The listing builds one solid part. Answer for the finished solid, in the listing's coordinates (mm). Face numbers are marked on the shaded views. A direction names the side the tool comes from. Coordinates: 2 decimals unless noted, no trailing zeros. Order: outer loops, then holes, each group sorted by start corner. A loop starts at its lowest first (then second) coordinate and runs counter-clockwise, first axis right, second up. Notation, with made-up numbers: (14.25, 28.25) -> (45.25, 28.25) arc R28 ccw to (45.25, 65.25) -> close; hole circle Ø2 at (60, 23.5). An arc over 180 degrees is marked (long way). Answer in a Markdown table with one row per item.
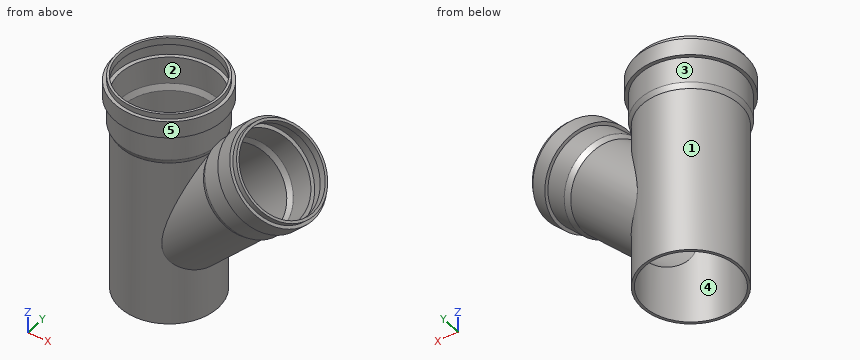
Autodesk Inventor part; units mm, degrees
ref_plane "YZ Plane" through (0, 0, 0) normal (1, 0, 0) x (0, 1, 0)
ref_plane "XZ Plane" through (0, 0, 0) normal (0, 1, 0) x (-1, 0, 0)
ref_plane "XY Plane" through (0, 0, 0) normal (0, 0, 1) x (1, 0, 0)
sketch "Sketch1" plane through (0, 0, 0) normal (0, 1, 0) x (-1, 0, 0)
  line L0 (0, 0) -> (0, 283.8404)
  line L1 (-65.58, 222.1797) -> (-62.5, 215.8203)
  line L2 (-65.58, 283.8404) -> (-62.7, 283.8404)
  line L3 (-62.7, 222.8404) -> (-59.3, 215.8203)
  line L4 (0, 0) -> (-62.5, 0) construction
  line L5 (-59.3, 215.8203) -> (-59.3, 0)
  line L6 (-62.5, 215.8203) -> (-62.5, 0)
  line L7 (-59.3, 0) -> (-62.5, 0)
  line L8 (-62.7, 283.8404) -> (0, 283.8404) construction
  line L9 (-62.5, 0) -> (-59.3, 0)
  line L10 (-64.04, 219) -> (0, 219) construction
  line L11 (0, 78) -> (-62.5, 78) construction
  line L12 (0, 60) -> (-62.5, 60) construction
  line L13 (0, 78) -> (-145.3176, 223.3176)
  line L14 (0, 78) -> (-36.6281, 41.3719) construction
  line L15 (-36.6281, 41.3719) -> (-135.9695, 140.7133)
  line L16 (-36.6281, 41.3719) -> (-38.8909, 39.1091) construction
  line L17 (-38.8909, 39.1091) -> (-138.2323, 138.4505)
  line L18 (-36.6281, 41.3719) -> (-38.8909, 39.1091)
  line L19 (-135.9695, 140.7133) -> (-143.3377, 143.2731)
  line L20 (-184.3499, 184.2853) -> (-186.6126, 182.0225)
  line L21 (-145.6004, 141.0103) -> (-138.2323, 138.4505)
  line L22 (-141.9163, 139.7304) -> (-101.8234, 179.8234) construction
  line L23 (-65.58, 222.1797) -> (-65.58, 255.4404)
  line L24 (-65.58, 255.4404) -> (-69.9, 255.4404)
  line L25 (-69.9, 255.4404) -> (-69.9, 277.1404)
  line L26 (-69.9, 277.1404) -> (-65.58, 277.1404)
  line L27 (-65.58, 277.1404) -> (-65.58, 283.8404)
  line L28 (-62.7, 283.8404) -> (-62.7, 274.7404)
  line L29 (-62.7, 274.7404) -> (-67.5, 274.7404)
  line L30 (-67.5, 274.7404) -> (-67.5, 257.8404)
  line L31 (-67.5, 257.8404) -> (-62.7, 257.8404)
  line L32 (-62.7, 257.8404) -> (-62.7, 222.8404)
  line L33 (-143.3377, 143.2731) -> (-165.9651, 165.9005)
  line L34 (-165.9651, 165.9005) -> (-169.3592, 162.5064)
  line L35 (-169.3592, 162.5064) -> (-181.3093, 174.4565)
  line L36 (-181.3093, 174.4565) -> (-177.9152, 177.8506)
  line L37 (-184.3499, 184.2853) -> (-177.9152, 177.8506)
  line L38 (-186.6126, 182.0225) -> (-181.875, 177.2849)
  line L39 (-181.875, 177.2849) -> (-184.7034, 174.4565)
  line L40 (-184.7034, 174.4565) -> (-169.3592, 159.1123)
  line L41 (-169.3592, 159.1123) -> (-166.5308, 161.9407)
  line L42 (-166.5308, 161.9407) -> (-145.6004, 141.0103)
  line L43 (-184.3499, 184.2853) -> (-145.3176, 223.3176) construction
  line L44 (-135.9695, 140.7133) -> (-99.3414, 177.3414) construction
  line L45 (-143.3377, 143.2731) -> (-104.3054, 182.3054) construction
  line L46 (-62.5, 215.8203) -> (-59.3, 215.8203) construction
  line L47 (-62.7, 222.8404) -> (0, 222.8404) construction
  dimension "d0" = 125
  dimension "d1" = 3.2
  dimension "d2" = 60
  dimension "d3" = 18
  dimension "d4" = 141
  dimension "d5" = 45
  dimension "d6" = 110
  dimension "d7" = 3.2
  dimension "d8" = 144
  dimension "d12" = 125.4
  dimension "d13" = 2.4
  dimension "d14" = 2.4
  dimension "d15" = 2.4
  dimension "d16" = 26
  dimension "d17" = 7.2
  dimension "d18" = 2.88
  dimension "d19" = 2.4
  dimension "d20" = 2.4
  dimension "d21" = 2.4
  dimension "d22" = 7.2
  dimension "d23" = 26
  dimension "d24" = 110.4
  dimension "d25" = 9.1
  dimension "d26" = 2.88
  dimension "d27" = 35
  dimension "d28" = 2.88
  dimension "d29" = 9.1
  dimension "d30" = 32
revolve "Revolution1" add sketch "Sketch1" angle 360 about axis through (0, 0, 0) along (0, 0, 1) contours L23 L24 L25 L26 L27 L2 L28 L29 L30 L31 L32 L3 L5 L13 L6 L1 | L13 L5 L15 L6 | L15 L5 L17 L6 | L17 L5 L7 L6
revolve "Revolution2" add sketch "Sketch1" angle 360 about axis through (0, 0, 78) along (0.7071, 0, 0.7071) contours L15 L5 L17 L6 | L6 L17 L21 L42 L41 L40 L39 L38 L20 L37 L36 L35 L34 L33 L19 L15 | L15 L18 L17 L5
sketch "Sketch2" plane through (145.3176, 0, 223.3176) normal (0.7071, 0, 0.7071) x (0.7071, 0, -0.7071)
  circle A0 centre (0, 0) radius 55.2
  circle A1 centre (0, 0) radius 51.8
  arc A2 (-16.8261, -2.4255) -> (-16.8261, 2.4255) centre (0, 0) ccw
sketch "Sketch3" plane through (0, 0, 283.8404) normal (0, 0, 1) x (1, 0, 0)
  circle A0 centre (0, 0) radius 62.7
  circle A1 centre (0, 0) radius 59.3
  arc A2 (34.4837, 1.0611) -> (34.4837, -1.0611) centre (0, 0) ccw
extrude "Extrusion1" cut sketch "Sketch3" against normal through all contours A1
extrude "Extrusion2" cut sketch "Sketch2" against normal up to surface contours A1
equation "\"d0\" = De"
equation "\"d2\" = L1"
equation "\"d3\" = z1"
equation "\"d12\" = Ds"
equation "\"d13\" = e3"
equation "\"d10\" = L1 + z2"
equation "\"De\" = 125"
equation "\"Ds\" = 125.4"
equation "\"L1\" = 60"
equation "\"e\" = 3.2"
equation "\"z1\" = 18"
equation "\"z2\" = 144"
equation "\"z3\" = 141"
equation "\"e2\" = 0.9 * e"
equation "\"e3\" = 0.75 * e"
equation "\"A\" = 35"
equation "\"C1\" = 26"
equation "\"C2\" = 26"
equation "\"A1\" = 32"
equation "\"e1\" = 3.2"
equation "\"e12\" = 2.88"
equation "\"e13\" = 2.4"
equation "\"L2\" = 54"
equation "\"Ds1\" = 110.4"
equation "\"Size_Designation\" = 1.2345"
properties part number "ISO 3633 45 Deg Reducing Branch with Single Socket for Elastomeric Sealing Ring Joints DN125 x DN110" material "PVC, Unplasticized"
(1) Which of the six approach directions +Z, -Z, +X, -X, +Y, -Y give full straight-line access (tool end or side, diameter ignored) to the marked faces 3, 4 and 5?
Check values:
| item | result |
|---|---|
| face 3 | none |
| face 4 | +Z, -Z |
| face 5 | +Z |
(2) For a pull along Y with two mould halves and no side action, classify the marked faces 1 and 2 as released by +Y, released by -Y, zero draft, split by the parting line, or undercut.
Check values:
| item | result |
|---|---|
| face 1 | split by the parting line |
| face 2 | undercut |
(3) Find the intervals of material crossed by line 1 along Y through (x, z) = (0, 265); line 2 along Y through (x, z) = (0, 246.5); line 3 along Z through (x, y) = (59.5, 27), in increasing order. Write a range as from..to.
Check values:
| item | result |
|---|---|
| line 1 | -69.9..-67.5, 67.5..69.9 |
| line 2 | -65.58..-62.7, 62.7..65.58 |
| line 3 | 69.74..74.98, 200.02..205.26, 221.68..257.84, 274.74..283.84 |
(4) Flat-ended cylindrical pins translate along their axes: pin 1 (2 mm diameter, centred on x = 9, z = 170.5, fed in from +Y); pin 2 (10 mm diameter, centred on y = 23, z = 213, fed in from +X); pin 3 (2 mm diameter, centred on y = 53, z = 76.5, fed in from +X). Find the tip coordinate at first contact, or state that the pin passes through.
Check values:
| item | result |
|---|---|
| pin 1 | y = 61.99 |
| pin 2 | x = 70.19 |
| pin 3 | x = 34.67 |
(5) A cutting plane is placed at C-C, the plane y = 40. Count the separate pieces of the cut face and the enclosed holes in it, then the cut area to 3 significant figures.
Check values:
| item | result |
|---|---|
| separate pieces | 3 |
| enclosed holes | 0 |
| area | 3,270 mm² |
(6) A cutting plane is placed at B-B, the plane z = 22.5. Determine the outline of the cut face in (x, y).
Check values:
| item | result |
|---|---|
| outline | circle Ø125 at (0, 0); hole circle Ø118.6 at (0, 0) |
